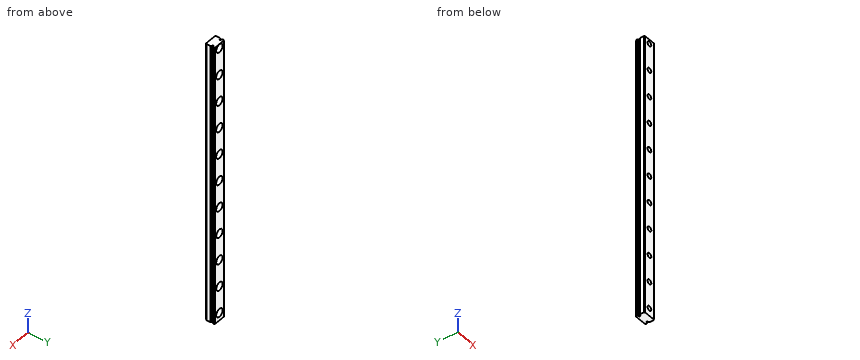
from build123d import *

# Parameters (mm, degrees)
BOSS_EXTRUDE1_DEPTH = 208.9
SKETCH2_R           = 3
CUT_EXTRUDE1_DEPTH  = 3.5
SKETCH3_R           = 1.75
CUT_EXTRUDE2_DEPTH  = 4


with BuildPart() as part:
    # Sketch1 → Boss-Extrude1 (new body)
    with BuildSketch(Plane.XY):
        with BuildLine():
            Line((-4.1, 6.5), (-4.5, 6.1))
            Line((-4.5, 6.1), (-4.5, 5.411997899))
            ThreePointArc((-4.5, 5.411997899), (-4.481535993, 5.345216747), (-4.431388889, 5.297405559))
            ThreePointArc((-4.431388889, 5.297405559), (-4.224528747, 5.147646302), (-4.065036084, 4.948194444))
            ThreePointArc((-4.065036084, 4.948194444), (-4.01760557, 4.901896679), (-3.953514706, 4.885))
            Line((-3.953514706, 4.885), (-3.688448805, 4.885))
            ThreePointArc((-3.688448805, 4.885), (-3.669364148, 4.886408492), (-3.650693039, 4.890603448))
            ThreePointArc((-3.650693039, 4.890603448), (-3.07, 4.46), (-3.650693039, 4.029396552))
            ThreePointArc((-3.650693039, 4.029396552), (-3.669364148, 4.033591508), (-3.688448805, 4.035))
            Line((-3.688448805, 4.035), (-3.953514706, 4.035))
            ThreePointArc((-3.953514706, 4.035), (-4.01760557, 4.018103321), (-4.065036084, 3.971805556))
            ThreePointArc((-4.065036084, 3.971805556), (-4.224528747, 3.772353698), (-4.431388889, 3.622594441))
            ThreePointArc((-4.431388889, 3.622594441), (-4.481535993, 3.574783253), (-4.5, 3.508002101))
            Line((-4.5, 3.508002101), (-4.5, 0.4))
            Line((-4.5, 0.4), (-4.1, 0))
            Line((-4.1, 0), (4.1, 0))
            Line((4.1, 0), (4.5, 0.4))
            Line((4.5, 0.4), (4.5, 3.508002101))
            ThreePointArc((4.5, 3.508002101), (4.481535993, 3.574783253), (4.431388889, 3.622594441))
            ThreePointArc((4.431388889, 3.622594441), (4.224528747, 3.772353698), (4.065036084, 3.971805556))
            ThreePointArc((4.065036084, 3.971805556), (4.01760557, 4.018103321), (3.953514706, 4.035))
            Line((3.953514706, 4.035), (3.688448805, 4.035))
            ThreePointArc((3.688448805, 4.035), (3.669364148, 4.033591508), (3.650693039, 4.029396552))
            ThreePointArc((3.650693039, 4.029396552), (3.07, 4.46), (3.650693039, 4.890603448))
            ThreePointArc((3.650693039, 4.890603448), (3.669364148, 4.886408492), (3.688448805, 4.885))
            Line((3.688448805, 4.885), (3.953514706, 4.885))
            ThreePointArc((3.953514706, 4.885), (4.01760557, 4.901896679), (4.065036084, 4.948194444))
            ThreePointArc((4.065036084, 4.948194444), (4.224528747, 5.147646302), (4.431388889, 5.297405559))
            ThreePointArc((4.431388889, 5.297405559), (4.481535993, 5.345216747), (4.5, 5.411997899))
            Line((4.5, 5.411997899), (4.5, 6.1))
            Line((4.5, 6.1), (4.1, 6.5))
            Line((4.1, 6.5), (-4.1, 6.5))
        make_face()
    extrude(amount=BOSS_EXTRUDE1_DEPTH)

    # Sketch2 → Cut-Extrude1 (cut)
    with BuildSketch(Plane(origin=(0, 6.5, 0), x_dir=(1, 0, 0), z_dir=(0, 1, 0))):
        with Locations((0, -205.7)):
            Circle(SKETCH2_R)
        with Locations((0, -185.7)):
            Circle(SKETCH2_R)
        with Locations((0, -165.7)):
            Circle(SKETCH2_R)
        with Locations((0, -145.7)):
            Circle(SKETCH2_R)
        with Locations((0, -125.7)):
            Circle(SKETCH2_R)
        with Locations((0, -105.7)):
            Circle(SKETCH2_R)
        with Locations((0, -85.7)):
            Circle(SKETCH2_R)
        with Locations((0, -65.7)):
            Circle(SKETCH2_R)
        with Locations((0, -45.7)):
            Circle(SKETCH2_R)
        with Locations((0, -25.7)):
            Circle(SKETCH2_R)
        with Locations((0, -5.7)):
            Circle(SKETCH2_R)
    extrude(amount=-CUT_EXTRUDE1_DEPTH, mode=Mode.SUBTRACT)

    # Sketch3 → Cut-Extrude2 (cut, through all)
    with BuildSketch(Plane(origin=(0, 3, 0), x_dir=(1, 0, 0), z_dir=(0, 1, 0))):
        with Locations((0, -205.7)):
            Circle(SKETCH3_R)
        with Locations((0, -185.7)):
            Circle(SKETCH3_R)
        with Locations((0, -165.7)):
            Circle(SKETCH3_R)
        with Locations((0, -145.7)):
            Circle(SKETCH3_R)
        with Locations((0, -125.7)):
            Circle(SKETCH3_R)
        with Locations((0, -105.7)):
            Circle(SKETCH3_R)
        with Locations((0, -85.7)):
            Circle(SKETCH3_R)
        with Locations((0, -65.7)):
            Circle(SKETCH3_R)
        with Locations((0, -45.7)):
            Circle(SKETCH3_R)
        with Locations((0, -25.7)):
            Circle(SKETCH3_R)
        with Locations((0, -5.7)):
            Circle(SKETCH3_R)
        with Locations((0, 14.3)):
            Circle(SKETCH3_R)
    extrude(amount=-CUT_EXTRUDE2_DEPTH, mode=Mode.SUBTRACT)


solid = part.part
The model under review builds one solid part; all positions refer to its coordinate system, in mm. Round coordinates to 2 decimals unless told otherwise and drop trailing zeros. Answer as CSV lines item,"result".
1. To check wall thickness, follow L1, parallel to X at y = 1.85, z = 105.7; L2, parallel to Y at x = 4, z = 141; L3, parallel to X at y = 5.3, z = 165.7. State the ranges of each line that lie inside material, in increasing order. Write a range as [from, to].
Outcome:
L1,"x = [-4.5, -1.75], [1.75, 4.5]"
L2,"y = [0, 4.03], [4.89, 6.5]"
L3,"x = [-4.44, -3], [3, 4.44]"
2. Insertion check: pin 1 Ø1.8 at (x, z) = (1, 104.5) entering from +Y; pin 2 Ø3 at (x, z) = (0, 205.7) entering from -Y. Each pin has a flat end and moves straight along its axis. Give the tip position at first contact, or say it passes through.
Outcome:
pin 1,"stops at y = 3"
pin 2,"passes through"
3. We need section B-B (x = 0). Count the separate pieces of the cut face and the enclosed holes in it, plus the area to 3 significant figures.
Outcome:
separate pieces,"12"
enclosed holes,"0"
area,"1,010 mm2"
